from build123d import *

# Parameters (mm, degrees)
CUT_EXTRUDE1_DEPTH = 1.8


with BuildPart() as part:
    # Sketch1 → Revolve1 (revolve)
    with BuildSketch(Plane.XY, mode=Mode.PRIVATE) as revolve1_sk:
        Polygon((0, 0), (0, 3), (5, 3), (5, 4), (6, 4), (6, 3), (14, 3), (14, 0), align=None)
    revolve(revolve1_sk.sketch.rotate(Axis((0, 0, 0), (1, 0, 0)), 180), axis=Axis((0, 0, 0), (1, 0, 0)))

    # Sketch2 → Cut-Revolve1 (revolve, cut)
    with BuildSketch(Plane.XY, mode=Mode.PRIVATE) as cut_revolve1_sk:
        Polygon((0, 0), (0, 1.5), (1.8, 1.5), (2.666025404, 0), align=None)
    revolve(cut_revolve1_sk.sketch.rotate(Axis((0, 0, 0), (1, 0, 0)), 90), axis=Axis((0, 0, 0), (1, 0, 0)), mode=Mode.SUBTRACT)

    # Sketch3 → Cut-Extrude1 (cut)
    with BuildSketch(Plane.ZY):
        Polygon((0, 1.732050808), (-1.5, 0.866025404), (-1.5, -0.866025404), (0, -1.732050808), (1.5, -0.866025404), (1.5, 0.866025404), align=None)
    extrude(amount=-CUT_EXTRUDE1_DEPTH, mode=Mode.SUBTRACT)


solid = part.part
Geometry: final body of the model. Coordinates: model frame, mm. A direction names the side the tool comes from. Give positions to 0.01 mm unless a question says otherwise; leave off trailing zeros. Write each loop counter-clockwise with the first axis right and the second up, starting at its lowest first coordinate (ties: lowest second). Pieces come first, ordered by that corner, then holes. Notation, with made-up numbers: (-14, 38) -> (-2, 38) arc R14 ccw to (-2, 63) -> close; hole circle Ø4 at (53.25, -17.5). An arc over 180 degrees is marked (long way). Answer as a JSON object with one key per item and string values.
1. Ray query, probe 1 along X at (y, z) = (3, 1); probe 2 along Z at (x, y) = (1, 0.5); probe 3 along Z at (x, y) = (3, 0). Return the intervals inside material, ascending. Write a range as from..to.
Ans:
{"probe 1": "x = 5..6", "probe 2": "z = -2.96..-1.5, 1.5..2.96", "probe 3": "z = -3..3"}
2. Contact query for flat-ended pins moving along their axis: pin 1 (3 mm diameter, centred on x = 7, y = 2, fed in from +Z); pin 2 (1 mm diameter, centred on x = 1.5, y = -0.5, fed in from +Z); pin 3 (2 mm diameter, centred on x = 11, z = 2, fed in from -Y); pin 4 (1.5 mm diameter, centred on y = -0.5, z = 2.5, fed in from -X). Output: stop coordinate, or through.
Ans:
{"pin 1": "stops at z = 3.9", "pin 2": "stops at z = 3", "pin 3": "stops at y = -2.83", "pin 4": "stops at x = 0"}
3. Cut plane B-B on x = 5.5. Output: boundary loops of the cut face in (y, z).
Ans:
{"outline": "circle Ø8 at (0, 0)"}
4. Cut plane A-A on z = -2. Output: boundary loops of the cut face in (x, y), and give its area (3 significant figures).
Ans:
{"outline": "(0, -2.24) -> (5, -2.24) -> (5, -3.46) -> (6, -3.46) -> (6, -2.24) -> (14, -2.24) -> (14, 2.24) -> (6, 2.24) -> (6, 3.46) -> (5, 3.46) -> (5, 2.24) -> (0, 2.24) -> close", "area": "65.1 mm^2"}
5. Access query for faces 4 (the flat face through (0, 1.3, 1.3)), 5 (the flat face through (6, -1, -3)), 6 (the flat face through (0.887, 1.293, 0.76)). Directions: +Z, -Z, +X, -X, +Y, -Y. A direction counts if a zero-diameter tool reaches every point of the face in a straight line with its end or side. Return the directions, or none.
Ans:
{"face 4": "+Z, -Z, -X, +Y, -Y", "face 5": "+X", "face 6": "-X"}
6. Cut plane D-D on x = 8.5. Output: boundary loops of the cut face in (y, z), and give its area (3 significant figures).
Ans:
{"outline": "circle Ø6 at (0, 0)", "area": "28.3 mm^2"}
7. Mould query, pull axis Z, two halves, no side actions, for faces 1 (the flat face through (1, 0, -1.5)), 2 (the flat face through (14, 0, 0)), 3 (the cylindrical face through (2.54, -2.86, -0.9)). Classes: pulls with the +Z half, pulls with the -Z half, needs draft (parallel to the pull), parting line crosses it, or undercut.
Ans:
{"face 1": "undercut", "face 2": "needs draft", "face 3": "parting line crosses it"}
